Geometry check sheet. Reference: the model listing, model coordinates, mm. Coordinates: 2 decimals unless noted, no trailing zeros. Order: outer loops, then holes, each group sorted by start corner. A loop starts at its lowest first (then second) coordinate and runs counter-clockwise, first axis right, second up. Notation, with made-up numbers: (55, 31.25) -> (72, 31.25) arc R30 cw to (72, 59.25) -> close; hole circle Ø6 at (-25, 16). An arc over 180 degrees is marked (long way). Answer as CSV lines item,"result". Start each with the question number.
from build123d import *
from build123d.topology import SkipClean

# Parameters (mm, degrees)
SKETCH1_W                      = 390
SKETCH1_H                      = 3
BOSS_EXTRUDE1_DEPTH            = 5
DRAFT1_ANGLE                   = -15
CIRPATTERN1_COUNT              = 12
DRAFT1_OF_CIRPATTERN1_2_ANGLE  = -15
DRAFT1_OF_CIRPATTERN1_3_ANGLE  = -15
DRAFT1_OF_CIRPATTERN1_4_ANGLE  = -15
DRAFT1_OF_CIRPATTERN1_5_ANGLE  = -15
DRAFT1_OF_CIRPATTERN1_6_ANGLE  = -15
DRAFT1_OF_CIRPATTERN1_7_ANGLE  = -15
DRAFT1_OF_CIRPATTERN1_8_ANGLE  = -15
DRAFT1_OF_CIRPATTERN1_9_ANGLE  = -15
DRAFT1_OF_CIRPATTERN1_10_ANGLE = -15
DRAFT1_OF_CIRPATTERN1_11_ANGLE = -15
DRAFT1_OF_CIRPATTERN1_12_ANGLE = -15
CUT_EXTRUDE1_DEPTH             = 563.983125857


# Read off the part's stored shape, not the designer's step: CSK for M4 Countersunk Flat Head Screw1
with BuildPart() as part:
    # Sketch1 → Revolve1 (revolve)
    with BuildSketch(Plane.XY, mode=Mode.PRIVATE) as revolve1_sk:
        with Locations((355, 83.5)):
            Rectangle(SKETCH1_W, SKETCH1_H)
    revolve(revolve1_sk.sketch.rotate(Axis((0, 0, 0), (1, 0, 0)), 90), axis=Axis((0, 0, 0), (1, 0, 0)))

    # Sketch2 → Boss-Extrude1 (add, symmetric)
    with BuildSketch(Plane(origin=(155, 0, 0), x_dir=(0, 0, -1), z_dir=(1, 0, 0))):
        with BuildLine():
            Line((10.703147762, 81.298478633), (11.094726339, 84.272813217))
            ThreePointArc((11.094726339, 84.272813217), (0, 85), (-11.094726339, 84.272813217))
            Line((-11.094726339, 84.272813217), (-10.703147762, 81.298478633))
            ThreePointArc((-10.703147762, 81.298478633), (0, 82), (10.703147762, 81.298478633))
        make_face()
    boss_extrude1 = extrude(amount=BOSS_EXTRUDE1_DEPTH, both=True)

    # Draft1
    draft1_faces = [part.faces().sort_by_distance(p)[0] for p in [
        (155, 82.785645925, 10.89893705),
        (155, 82.785645925, -10.89893705),
    ]]
    draft(draft1_faces, Plane(origin=(155, 0, 0), x_dir=(0, 0, 1), z_dir=(1, 0, 0)), DRAFT1_ANGLE)

    # CirPattern1: Boss-Extrude1 ×12 about axis
    with SkipClean():  # the faces are left unmerged after this step: merging them gives an invalid solid
        cirpattern1_axis = Axis((0, 0, 0), (1, 0, 0))
        for i in range(1, CIRPATTERN1_COUNT):
            add(boss_extrude1.rotate(cirpattern1_axis, i * 360 / CIRPATTERN1_COUNT))

    # Draft1 of CirPattern1 2
    draft1_of_cirpattern1_2_faces = [part.faces().sort_by_distance(p)[0] for p in [
        (155, 66.245003914, 50.831579322),
        (155, 77.143940965, 31.954066602),
    ]]
    draft(draft1_of_cirpattern1_2_faces, Plane(origin=(155, 0, 0), x_dir=(0, -0.49999999999999994, 0.8660254037844387), z_dir=(1, 0, 0)), DRAFT1_OF_CIRPATTERN1_2_ANGLE)

    # Draft1 of CirPattern1 3
    draft1_of_cirpattern1_3_faces = [part.faces().sort_by_distance(p)[0] for p in [
        (155, 31.954066602, 77.143940965),
        (155, 50.831579322, 66.245003914),
    ]]
    draft(draft1_of_cirpattern1_3_faces, Plane(origin=(155, 0, 0), x_dir=(0, -0.8660254037844386, 0.5000000000000001), z_dir=(1, 0, 0)), DRAFT1_OF_CIRPATTERN1_3_ANGLE)

    # Draft1 of CirPattern1 4
    draft1_of_cirpattern1_4_faces = [part.faces().sort_by_distance(p)[0] for p in [
        (155, -10.89893705, 82.785645925),
        (155, 10.89893705, 82.785645925),
    ]]
    draft(draft1_of_cirpattern1_4_faces, Plane(origin=(155, 0, 0), x_dir=(0, -1, 0), z_dir=(1, 0, 0)), DRAFT1_OF_CIRPATTERN1_4_ANGLE)

    # Draft1 of CirPattern1 5
    draft1_of_cirpattern1_5_faces = [part.faces().sort_by_distance(p)[0] for p in [
        (155, -50.831579322, 66.245003914),
        (155, -31.954066602, 77.143940965),
    ]]
    draft(draft1_of_cirpattern1_5_faces, Plane(origin=(155, 0, 0), x_dir=(0, -0.8660254037844387, -0.4999999999999998), z_dir=(1, 0, 0)), DRAFT1_OF_CIRPATTERN1_5_ANGLE)

    # Draft1 of CirPattern1 6
    draft1_of_cirpattern1_6_faces = [part.faces().sort_by_distance(p)[0] for p in [
        (155, -77.143940965, 31.954066602),
        (155, -66.245003914, 50.831579322),
    ]]
    draft(draft1_of_cirpattern1_6_faces, Plane(origin=(155, 0, 0), x_dir=(0, -0.49999999999999994, -0.8660254037844387), z_dir=(1, 0, 0)), DRAFT1_OF_CIRPATTERN1_6_ANGLE)

    # Draft1 of CirPattern1 7
    draft1_of_cirpattern1_7_faces = [part.faces().sort_by_distance(p)[0] for p in [
        (155, -82.785645925, -10.89893705),
        (155, -82.785645925, 10.89893705),
    ]]
    draft(draft1_of_cirpattern1_7_faces, Plane(origin=(155, 0, 0), x_dir=(0, 0, -1), z_dir=(1, 0, 0)), DRAFT1_OF_CIRPATTERN1_7_ANGLE)

    # Draft1 of CirPattern1 8
    draft1_of_cirpattern1_8_faces = [part.faces().sort_by_distance(p)[0] for p in [
        (155, -66.245003914, -50.831579322),
        (155, -77.143940965, -31.954066602),
    ]]
    draft(draft1_of_cirpattern1_8_faces, Plane(origin=(155, 0, 0), x_dir=(0, 0.5000000000000001, -0.8660254037844386), z_dir=(1, 0, 0)), DRAFT1_OF_CIRPATTERN1_8_ANGLE)

    # Draft1 of CirPattern1 9
    draft1_of_cirpattern1_9_faces = [part.faces().sort_by_distance(p)[0] for p in [
        (155, -31.954066602, -77.143940965),
        (155, -50.831579322, -66.245003914),
    ]]
    draft(draft1_of_cirpattern1_9_faces, Plane(origin=(155, 0, 0), x_dir=(0, 0.8660254037844384, -0.5000000000000004), z_dir=(1, 0, 0)), DRAFT1_OF_CIRPATTERN1_9_ANGLE)

    # Draft1 of CirPattern1 10
    draft1_of_cirpattern1_10_faces = [part.faces().sort_by_distance(p)[0] for p in [
        (155, 10.89893705, -82.785645925),
        (155, -10.89893705, -82.785645925),
    ]]
    draft(draft1_of_cirpattern1_10_faces, Plane.YZ.offset(155), DRAFT1_OF_CIRPATTERN1_10_ANGLE)

    # Draft1 of CirPattern1 11
    draft1_of_cirpattern1_11_faces = [part.faces().sort_by_distance(p)[0] for p in [
        (155, 50.831579322, -66.245003914),
        (155, 31.954066602, -77.143940965),
    ]]
    draft(draft1_of_cirpattern1_11_faces, Plane(origin=(155, 0, 0), x_dir=(0, 0.8660254037844386, 0.5000000000000001), z_dir=(1, 0, 0)), DRAFT1_OF_CIRPATTERN1_11_ANGLE)

    # Draft1 of CirPattern1 12
    draft1_of_cirpattern1_12_faces = [part.faces().sort_by_distance(p)[0] for p in [
        (155, 77.143940965, -31.954066602),
        (155, 66.245003914, -50.831579322),
    ]]
    draft(draft1_of_cirpattern1_12_faces, Plane(origin=(155, 0, 0), x_dir=(0, 0.5000000000000004, 0.8660254037844384), z_dir=(1, 0, 0)), DRAFT1_OF_CIRPATTERN1_12_ANGLE)

    # Sketch3 → Cut-Extrude1 (cut, through all)
    with BuildSketch(Plane(origin=(0, 0, 0), x_dir=(0, 0, -1), z_dir=(1, 0, 0))):
        with BuildLine():
            Line((0, 0), (-85, 0))
            ThreePointArc((-85, 0), (0, 85), (85, 0))
            Line((85, 0), (0, 0))
        make_face()
    extrude(amount=CUT_EXTRUDE1_DEPTH, mode=Mode.SUBTRACT)

    # CSK for M4 Countersunk Flat Head Scr 2 → CSK for M4 Countersunk Flat Head Screw1 (revolve, cut)
    with BuildSketch(Plane(origin=(540, 0, 0), x_dir=(1, 0, 0), z_dir=(0, 0, 1))):
        Polygon((0, -85.000032153), (4.700032153, -85.000032153), (2.25, -82.55), (2.25, -81.96910869), (0, -81.96910869), align=None)
    revolve(axis=Axis((540, 0, 0), (0, 1, 0)), mode=Mode.SUBTRACT)


solid = part.part
Q1. Thickness scan on L1, parallel to X at y = -82.15, z = 0; L2, parallel to Z at x = 532, y = -74.5; L3, parallel to Z at x = 277.5, y = -14.5. Record the ranges inside material, lowest first.
Q2. Go/stop test with flat-tipped pins: pin 1 Ø5 at (x, z) = (220.5, 26.5) entering from -Y; pin 2 Ø5 at (x, y) = (198.5, -71.5) entering from -Z; pin 3 Ø8.5 at (y, z) = (-78.5, 20.5) entering from -X; pin 4 Ø3.5 at (x, z) = (540, 0) entering from -Y. Record where each tip stops, or that it passes through.
Q3. Sectioned sample at A-A, the plane y = -44. Record the cut outline in (x, z).
Q4. Release check for a two-part mould opening along X. For faces 1 (the conical face through (537.6, -82.7, -0.1)), 2 (the flat face through (150, -72, 42)), 3 (the flat face through (550, -84, 0)) record: released by +X, released by -X, zero draft, split by the parting line, or undercut.
Q5. Sectioned sample at C-C, the plane z = 38. Record the cut outline in (x, y), then the cut area to 3 significant figures.
Q6. Sectioned sample at B-B, the plane x = 462. Record the cut outline in (y, z).
Geometry results:
1,L1,"x = 150 to 537.75, 542.25 to 550"
1,L2,"z = -40.92 to -34.26, 34.26 to 40.92"
1,L3,"z = -83.75 to -80.71, 80.71 to 83.75"
2,pin 1,"stops at y = -81.54"
2,pin 2,"stops at z = -49.64"
2,pin 3,"stops at x = 160"
2,pin 4,"passes through"
3,outline,"(150, -72.73) -> (550, -72.73) -> (550, -69.2) -> (150, -69.2) -> close; (150, 69.2) -> (550, 69.2) -> (550, 72.73) -> (150, 72.73) -> close"
4,face 1,"undercut"
4,face 2,"released by -X"
4,face 3,"released by +X"
5,outline,"(150, -76.03) -> (550, -76.03) -> (550, -72.66) -> (150, -72.66) -> close"
5,area,"1,350 mm^2"
6,outline,"(0, -85) -> (0, -82) arc R82 cw to (0, 82) -> (0, 85) arc R85 ccw to start"
